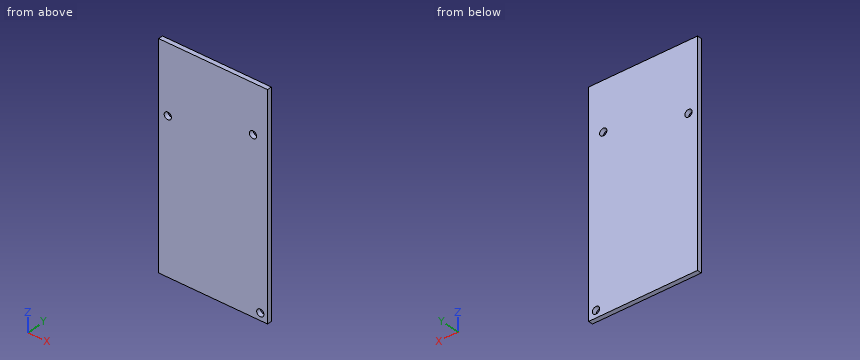
from build123d import *

# Parameters (mm, degrees)
SKETCH1_W                   = 38.1
SKETCH1_H                   = 93.98
BOSS_EXTRUDE1_DEPTH         = 1.6
CUT_EXTRUDE1_DEPTH          = 51.729898482
CUT_EXTRUDE1_DEPTH_BACK     = 51.729898482
SKETCH2_R                   = 1.27
CUT_EXTRUDE2_DEPTH          = 51.729898482
CUT_EXTRUDE2_DEPTH_BACK     = 51.729898482
SKETCH3_R                   = 1.27
SKETCH3_W                   = 38.1
SKETCH3_H                   = 16.505
BODY_MOVE_COPY1_DEPTH       = 1.6
BODY_MOVE_COPY1_2_OUTLINE_W = 38.1
BODY_MOVE_COPY1_2_OUTLINE_H = 16.505
BODY_MOVE_COPY1_2_OUTLINE_R = 1.27
BODY_MOVE_COPY1_2_DEPTH     = 1.6


# Read off the part's stored shape, not the designer's step: Body-Move/Copy1
with BuildPart() as part:
    # Sketch1 → Boss-Extrude1 (new body)
    with BuildSketch(Plane(origin=(0, 0, 0), x_dir=(1, 0, 0), z_dir=(0, 1, 0))):
        Rectangle(SKETCH1_W, SKETCH1_H)
    extrude(amount=BOSS_EXTRUDE1_DEPTH)

    # Sketch2 → Cut-Extrude1 (cut, two sides: drawn at the far end of the back side and taken through both)
    with BuildSketch(Plane(origin=(0, 1.6, 0), x_dir=(1, 0, 0), z_dir=(0, 1, 0)).offset(-CUT_EXTRUDE1_DEPTH_BACK)):
        with Locations(Location((13.97, -29.84, 0), (0, 0, 270))):
            Circle(SKETCH2_R)
        with Locations(Location((-15.875, -6.35, 0), (0, 0, 270))):
            Circle(SKETCH2_R)
        with Locations(Location((16.51, 44.45, 0), (0, 0, 270))):
            Circle(SKETCH2_R)
    extrude(amount=CUT_EXTRUDE1_DEPTH + CUT_EXTRUDE1_DEPTH_BACK, mode=Mode.SUBTRACT)

    # Sketch3 → Cut-Extrude2 (cut, two sides: drawn at the far end of the back side and taken through both)
    with BuildSketch(Plane(origin=(0, 1.6, 0), x_dir=(1, 0, 0), z_dir=(0, 1, 0)).offset(-CUT_EXTRUDE2_DEPTH_BACK)):
        with Locations(Location((-15.875, -6.35, 0), (0, 0, 270))):
            Circle(SKETCH3_R)
        with Locations((0, -18.5875)):
            Rectangle(SKETCH3_W, SKETCH3_H)
    extrude(amount=CUT_EXTRUDE2_DEPTH + CUT_EXTRUDE2_DEPTH_BACK, mode=Mode.SUBTRACT)


with BuildPart() as cut_extrude2_piece_1:
    # of the separate pieces the step leaves, piece 1, a body of its own (cut_extrude2_pieces)
    add(part.part.solids().sort_by_distance((-19.05, 0, -46.99))[0])


with BuildPart() as cut_extrude2_piece_2:
    # of the separate pieces the step leaves, piece 2, a body of its own (cut_extrude2_pieces)
    add(part.part.solids().sort_by_distance((-19.05, 0, 46.99))[0])

    # Body-Move/Copy1 outline → Body-Move/Copy1 (cut)
    with BuildSketch(Plane(origin=(0, 0, 0), x_dir=(1, 0, 0), z_dir=(0, 1, 0))):
        with BuildLine():
            Line((12.875982176, -30.485), (-19.05, -30.485))
            Line((-19.05, -30.485), (-19.05, -46.99))
            Line((-19.05, -46.99), (19.05, -46.99))
            Line((19.05, -46.99), (19.05, -30.485))
            Line((19.05, -30.485), (15.064017824, -30.485))
            ThreePointArc((15.064017824, -30.485), (13.97, -31.11), (12.875982176, -30.485))
        make_face()
    extrude(amount=BODY_MOVE_COPY1_DEPTH, mode=Mode.SUBTRACT)

    # Body-Move_Copy1 2 outline → Body-Move_Copy1 2 (add)
    # profile 1 of 2: a face of its own
    with BuildSketch(Plane(origin=(0, 0, 0), x_dir=(1, 0, 0), z_dir=(0, 1, 0))):
        with Locations((0, -18.5875)):
            Rectangle(BODY_MOVE_COPY1_2_OUTLINE_W, BODY_MOVE_COPY1_2_OUTLINE_H)
        with Locations((13.97, -13.335)):
            Circle(BODY_MOVE_COPY1_2_OUTLINE_R, mode=Mode.SUBTRACT)
    # profile 2 of 2: a face of its own
    with BuildSketch(Plane(origin=(0, 0, 0), x_dir=(1, 0, 0), z_dir=(0, 1, 0))):
        with BuildLine():
            ThreePointArc((15.064017824, -30.485), (13.97, -28.57), (12.875982176, -30.485))
            Line((12.875982176, -30.485), (15.064017824, -30.485))
        make_face()
    extrude(amount=BODY_MOVE_COPY1_2_DEPTH)

    # Combine1: union Cut-Extrude2 piece 1
    add(cut_extrude2_piece_1.part)


solid = cut_extrude2_piece_2.part
The model under review builds one solid part; all positions refer to its coordinate system, in mm. Give positions to 0.01 mm unless a question says otherwise; leave off trailing zeros. Loops run counter-clockwise (first coordinate to the right, second up) from the corner with the lowest first, then second, coordinate; pieces in that order, holes last. Notation, with made-up numbers: (78.5, 53) -> (120.5, 53) arc R31 ccw to (120.5, 90) -> close; hole circle Ø5 at (66, 64.25). An arc over 180 degrees is marked (long way). Answer as a JSON object with one key per item and string values. Group by question number.
Q1. Take a section at B-B (z = 6.35). Write out the cut boundary in (x, y) (3 decimals), plus the area to 3 significant figures.
Q2. Wall thickness on line 1 along X through (y, z) = (0.45, 6.35) (3 decimals); line 2 along Z through (x, y) = (16.51, 0.4) (3 decimals); line 3 along Z through (x, y) = (13.97, 0.7) (3 decimals): over which ranges is each line inside the solid? List them lowest first.
Q3. Insertion check: pin 1 (1.5 mm diameter, centred on x = 16.51, z = -44.45, fed in from -Y). The pin has a flat end and moves straight along its axis. Give the tip position at first contact, or say it passes through.
Q4. Take a section at A-A (x = 13.97). Write out the cut boundary in (y, z) (3 decimals), plus the area to 3 significant figures.
Answer below:
{
 "1": {"outline": "(-19.05, 0) -> (-17.145, 0) -> (-17.145, 1.6) -> (-19.05, 1.6) -> close; (-14.605, 0) -> (19.05, 0) -> (19.05, 1.6) -> (-14.605, 1.6) -> close", "area": "56.9 mm2"},
 "2": {"line 1": "x = -19.05 to -17.145, -14.605 to 19.05", "line 2": "z = -46.99 to -45.72, -43.18 to 30.485", "line 3": "z = -46.99 to 12.065, 14.605 to 30.485"},
 "3": {"pin 1": "passes through"},
 "4": {"outline": "(0, -46.99) -> (1.6, -46.99) -> (1.6, 12.065) -> (0, 12.065) -> close; (0, 14.605) -> (1.6, 14.605) -> (1.6, 30.485) -> (0, 30.485) -> close", "area": "120 mm2"}
}
